For this review, take the finished solid that the model builds, in its own axes (mm). A direction names the side the tool comes from. Give positions to 0.01 mm unless a question says otherwise; leave off trailing zeros. Order: outer loops, then holes, each group sorted by start corner. A loop starts at its lowest first (then second) coordinate and runs counter-clockwise, first axis right, second up. Notation, with made-up numbers: (-34.75, 45.5) -> (-6.75, 45.5) arc R12 cw to (-6.75, 67.5) -> close; hole circle Ø3 at (29.25, 79). An arc over 180 degrees is marked (long way). One line per item, written item: value. Start each with the question number.
Autodesk Inventor part; units mm, degrees
ref_plane "YZ Plane" through (0, 0, 0) normal (1, 0, 0) x (0, 1, 0)
ref_plane "XZ Plane" through (0, 0, 0) normal (0, 1, 0) x (-1, 0, 0)
ref_plane "XY Plane" through (0, 0, 0) normal (0, 0, 1) x (1, 0, 0)
sketch "Sketch2" plane through (0, 0, 0) normal (0, 1, 0) x (-1, 0, 0)
  line L0 (-40, 60) -> (40, 60)
  line L1 (40, 60) -> (40, -60)
  line L2 (40, -60) -> (-40, -60)
  line L3 (-40, -60) -> (-40, 60)
  line L4 (-40, 60) -> (40, -60) construction
  line L5 (40, 60) -> (-40, -60) construction
  line L6 (-37.76, 57.76) -> (37.76, 57.76)
  line L7 (37.76, 57.76) -> (37.76, -57.76)
  line L8 (37.76, -57.76) -> (-37.76, -57.76)
  line L9 (-37.76, -57.76) -> (-37.76, 57.76)
  line L10 (-37.76, 57.76) -> (37.76, -57.76) construction
  line L11 (37.76, 57.76) -> (-37.76, -57.76) construction
  point P0 (0, 0)
  dimension "d8" = 80
  dimension "d9" = 120
  dimension "d10" = 75.52
  dimension "d61" = 115.52
extrude "Extrusion2" add sketch "Sketch2" along normal mid plane 790
fillet "Fillet2" radius 4 4 edges at (-40, 0, 60) (40, 0, 60) (40, 0, -60) (-40, 0, -60)
fillet "Fillet2" radius 2 4 edges at (37.76, 0, 57.76) (-37.76, 0, -57.76) (37.76, 0, -57.76) (-37.76, 0, 57.76)
properties part number "tubo3-40x80x800" material "Acero, carbono"
Q1. Mouldability with a two-part tool opening along X and no side actions: class faces 1 (the flat face through (-37.76, -6, 1)), 2 (the flat face through (40, -6, -1)), 3 (the flat face through (-40, -6, 1)) as pulls with the +X half, pulls with the -X half, needs draft (parallel to the pull), parting line crosses it, or undercut.
Q2. Take a section at C-C (y = -96.5). State the section outline as (x, z) points.
Q3. For line 1 along X through (y, z) = (58, -45); line 2 along Z through (x, y) = (-21, 246.5), list the stretches that pass through material, from the lowest coordinate up.
Q4. Take a section at A-A (z = 49). State the section outline as (x, y) points.
Q5. For faces 4 (the flat face through (-38, 395, 18)), 5 (the flat face through (1, -6, 57.76)), list the 3-axis set-ups (+Z, -Z, +X, -X, +Y, -Y) from which the entire face can be reached by the end or side of a thin tool; tool diameter is ignored.
Q6. Take a section at B-B (x = -13). State the section outline as (y, z) points.
Answers below:
1. face 1: undercut
1. face 2: pulls with the +X half
1. face 3: pulls with the -X half
2. outline: (-40, -56) arc R4 ccw to (-36, -60) -> (36, -60) arc R4 ccw to (40, -56) -> (40, 56) arc R4 ccw to (36, 60) -> (-36, 60) arc R4 ccw to (-40, 56) -> close; hole (-37.76, -55.76) arc R2 ccw to (-35.76, -57.76) -> (35.76, -57.76) arc R2 ccw to (37.76, -55.76) -> (37.76, 55.76) arc R2 ccw to (35.76, 57.76) -> (-35.76, 57.76) arc R2 ccw to (-37.76, 55.76) -> close
3. line 1: x = -40 to -37.76, 37.76 to 40
3. line 2: z = -60 to -57.76, 57.76 to 60
4. outline: (-40, -395) -> (-37.76, -395) -> (-37.76, 395) -> (-40, 395) -> close; (37.76, -395) -> (40, -395) -> (40, 395) -> (37.76, 395) -> close
5. face 4: +Z, -Z, +X, -X, +Y
5. face 5: +Y, -Y
6. outline: (-395, -60) -> (395, -60) -> (395, -57.76) -> (-395, -57.76) -> close; (-395, 57.76) -> (395, 57.76) -> (395, 60) -> (-395, 60) -> close
